For this review, take the finished solid that the model builds, in its own axes (mm). A direction names the side the tool comes from. Give positions to 0.01 mm unless a question says otherwise; leave off trailing zeros. Write each loop counter-clockwise with the first axis right and the second up, starting at its lowest first coordinate (ties: lowest second). Pieces come first, ordered by that corner, then holes. Notation, with made-up numbers: M -17,8.5 L -6,8.5 A31 ccw -6,42.5 Z; hole C -18,14 d7. An arc over 180 degrees is marked long. One line per item, written item: value. Start each with the question number.
Item 1: To check wall thickness, follow probe 1 along X at (y, z) = (-15.1, 0); probe 2 along X at (y, z) = (-5.5, 0); probe 3 along Y at (x, z) = (-2, 2.5). State the ranges of each line that lie inside material, in increasing order.
Item 2: Consider section B-B, the plane z = 0. Write out the cut boundary in (x, y).
Item 3: Clearance check with flat-ended pins moving along their axes: pin 1 Ø1.5 at (x, y) = (2.5, -8) entering from +Z; pin 2 Ø2 at (x, y) = (-0.5, -2.5) entering from +Z; pin 3 Ø4 at (x, y) = (-1.5, -5) entering from -Z. State where each tip first meets the part, or that it passes through.
Item 4: Tool access review of faces 1 (the face through (1.5, -14, 0.7)), 2 (the face through (-3.905, -7.888, 0.867)), 3 (the face through (0.45, -15.01, -1.43)): name each direction out of +Z, -Z, +X, -X, +Y, -Y from which nothing blocks a thin tool from reaching the whole face with its end or side.
Item 5: Mouldability with a two-part tool opening along X and no side actions: class faces 4 (the face through (0, -16, -2)), 5 (the face through (-1.978, -5.888, -2.579)), 6 (the face through (-4.88, 0.99, -1.08)) as released by +X, released by -X, zero draft, split by the parting line, or undercut.
Item 6: Consider section C-C, the plane y = -5.5. Write out the cut boundary in (x, z), and give its area (3 significant figures).
Item 7: Consider section A-A, the plane x = 0. Write out the cut boundary in (y, z).
Item 8: Consider section D-D, the plane x = 3.5. Write out the cut boundary in (y, z).
```python
from build123d import *

# Parameters (mm, degrees)
SKIZZE1_R                       = 5
AUFSATZ_LINEAR_AUSTRAGEN1_DEPTH = 2
SKIZZE2_R                       = 4
AUFSATZ_LINEAR_AUSTRAGEN2_DEPTH = 16
SKIZZE3_R                       = 3.25
SCHNITT_LINEAR_AUSTRAGEN1_DEPTH = 16
SKIZZE4_R                       = 1.5
SCHNITT_LINEAR_AUSTRAGEN2_DEPTH = 2


with BuildPart() as part:
    # Skizze1 → Aufsatz-Linear austragen1 (new body)
    with BuildSketch(Plane(origin=(0, 0, 0), x_dir=(1, 0, 0), z_dir=(0, 1, 0))):
        with Locations(Location((0, 0, 0), (0, 0, 270))):
            Circle(SKIZZE1_R)
    extrude(amount=AUFSATZ_LINEAR_AUSTRAGEN1_DEPTH)

    # Skizze2 → Aufsatz-Linear austragen2 (add)
    with BuildSketch(Plane.XZ):
        with Locations(Location((0, 0, 0), (0, 0, 270))):
            Circle(SKIZZE2_R)
    extrude(amount=AUFSATZ_LINEAR_AUSTRAGEN2_DEPTH)

    # Skizze3 → Schnitt-Linear austragen1 (cut)
    with BuildSketch(Plane(origin=(0, 2, 0), x_dir=(1, 0, 0), z_dir=(0, 1, 0))):
        with Locations(Location((0, 0, 0), (0, 0, 270))):
            Circle(SKIZZE3_R)
    extrude(amount=-SCHNITT_LINEAR_AUSTRAGEN1_DEPTH, mode=Mode.SUBTRACT)

    # Skizze4 → Schnitt-Linear austragen2 (cut)
    with BuildSketch(Plane.XZ.offset(16)):
        with Locations(Location((0, 0, 0), (0, 0, 270))):
            Circle(SKIZZE4_R)
    extrude(amount=-SCHNITT_LINEAR_AUSTRAGEN2_DEPTH, mode=Mode.SUBTRACT)


solid = part.part
```
Model answer:
1. probe 1: x = -4 to -1.5, 1.5 to 4
1. probe 2: x = -4 to -3.25, 3.25 to 4
1. probe 3: y = -16 to -14
2. outline: M -5,0 L -4,0 L -4,-16 L -1.5,-16 L -1.5,-14 L -3.25,-14 L -3.25,2 L -5,2 Z; M 1.5,-16 L 4,-16 L 4,0 L 5,0 L 5,2 L 3.25,2 L 3.25,-14 L 1.5,-14 Z
3. pin 1: stops at z = 3.6
3. pin 2: stops at z = 4
3. pin 3: stops at z = -4
4. face 1: +Y
4. face 2: -Y
4. face 3: +Y, -Y
5. face 4: zero draft
5. face 5: undercut
5. face 6: split by the parting line
6. outline: C 0,0 d8; hole C 0,0 d6.5
6. area: 17.1 mm2
7. outline: M -16,-4 L 0,-4 L 0,-5 L 2,-5 L 2,-3.25 L -14,-3.25 L -14,-1.5 L -16,-1.5 Z; M -16,1.5 L -14,1.5 L -14,3.25 L 2,3.25 L 2,5 L 0,5 L 0,4 L -16,4 Z
8. outline: M -16,-1.94 L 0,-1.94 L 0,-3.57 L 2,-3.57 L 2,3.57 L 0,3.57 L 0,1.94 L -16,1.94 Z
